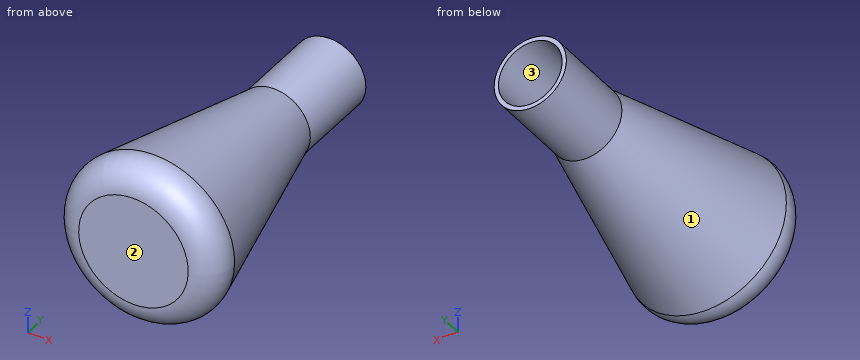
from build123d import *


with BuildPart() as part:
    # Croquis2 → Revolución1 (revolve)
    with BuildSketch(Plane.XY, mode=Mode.PRIVATE) as revoluci_n1_sk:
        with BuildLine():
            Line((17, 145), (17, 104))
            Line((17, 104), (37.898418039, 15.288347915))
            ThreePointArc((37.898418039, 15.288347915), (35.543424025, 4.716396984), (25.793155167, 0))
            Line((25.793155167, 0), (0, 0))
            Line((0, 0), (0, 2))
            Line((0, 2), (24.225162721, 2))
            ThreePointArc((24.225162721, 2), (33.380794894, 6.428759514), (35.592165604, 16.355962086))
            Line((35.592165604, 16.355962086), (15, 103.767603835))
            Line((15, 103.767603835), (15, 145))
            Line((15, 145), (17, 145))
        make_face()
    revolve(revoluci_n1_sk.sketch.rotate(Axis((0, 0, 0), (0, 1, 0)), 90), axis=Axis((0, 0, 0), (0, 1, 0)))


solid = part.part
Read the model definition and answer for the solid it produces. Units are mm, in the model's axes. Face numbers are marked on the shaded views. Round coordinates to 2 decimals unless told otherwise and drop trailing zeros. Write each loop counter-clockwise with the first axis right and the second up, starting at its lowest first coordinate (ties: lowest second). Pieces come first, ordered by that corner, then holes.
Q1. Find section D-D on y = 48. Determine the outline of the cut face in (x, z), and give its area (3 significant figures).
Values:
outline: circle Ø60.38 at (0, 0); hole circle Ø56.28 at (0, 0)
area: 377 mm2
Q2. Find section A-A on z = 0. Determine the outline of the cut face in (x, y).
Values:
outline: (-37.9, 15.29) arc R12.44 ccw to (-25.79, 0) - (25.79, 0) arc R12.44 ccw to (37.9, 15.29) - (17, 104) - (17, 145) - (15, 145) - (15, 103.77) - (35.59, 16.36) arc R11.68 cw to (24.23, 2) - (-24.23, 2) arc R11.68 cw to (-35.59, 16.36) - (-15, 103.77) - (-15, 145) - (-17, 145) - (-17, 104) - close
Q3. Flat-ended cylindrical pins translate along their axes: P1, Ø8, axis at y = 74, z = 6.5, coming from the +X side; P2, Ø8, axis at x = 15, y = 73, coming from the +Z side; P3, Ø4, axis at x = -7, y = 26, coming from the -Z side. Find the tip coordinate at first contact, or state that the pin passes through.
Values:
P1: stops at x = 24.48
P2: stops at z = 21.93
P3: stops at z = -35.28
Q4. Find section C-C on y = 88.5. Determine the outline of the cut face in (x, z), and give its area (3 significant figures).
Values:
outline: circle Ø41.3 at (0, 0); hole circle Ø37.19 at (0, 0)
area: 253 mm2
Q5. The mould has two halves that part along X. Classify the marked faces 1, 2 and 3: released by +X, released by -X, zero draft, split by the parting line, or undercut.
Values:
face 1: split by the parting line
face 2: zero draft
face 3: undercut
Q6. Find section B-B on x = 0. Determine the outline of the cut face in (y, z).
Values:
outline: (0, -25.79) arc R12.44 ccw to (15.29, -37.9) - (104, -17) - (145, -17) - (145, -15) - (103.77, -15) - (16.36, -35.59) arc R11.68 cw to (2, -24.23) - (2, 24.23) arc R11.68 cw to (16.36, 35.59) - (103.77, 15) - (145, 15) - (145, 17) - (104, 17) - (15.29, 37.9) arc R12.44 ccw to (0, 25.79) - close
Q7. Straight lines are drawn through the part: line 1 (X direction, y = 112.5, z = 0); line 2 (X direction, y = 22.5, z = 8); line 3 (Y direction, x = -1.5, z = -10.5). For each, find the intervals that lie inside material, in ascending order.
Values:
line 1: x = -17 to -15, 15 to 17
line 2: x = -35.3 to -33.19, 33.19 to 35.3
line 3: y = 0 to 2
